```python
from build123d import *

# Parameters (mm, degrees)
BASPROSKE_W             = 7
BASPROSKE_H             = 10.5
TOOTHCUT_DEPTH          = 17.416455159
TEETHCUTS_COUNT         = 12
TEETHCUTS_ANGLE         = 330
BORSKE_R                = 2.5
BORE_DEPTH              = 50.0000508
CROQUIS2_R              = 2.91
CORTAR_EXTRUIR1_DEPTH   = 11
CROQUIS3_R              = 3.252376505
CROQUIS3_R_2            = 1.9
SALIENTE_EXTRUIR2_DEPTH = 0.79


with BuildPart() as part:
    # BasProSke → Base-Revolve (revolve)
    with BuildSketch(Plane(origin=(0, 0, 0), x_dir=(1, 0, 0), z_dir=(0, 1, 0)), mode=Mode.PRIVATE) as base_revolve_sk:
        with Locations((3.5, 5.25)):
            Rectangle(BASPROSKE_W, BASPROSKE_H)
    revolve(base_revolve_sk.sketch.rotate(Axis((-10, 0, 0), (1, 0, 0)), 180), axis=Axis((-10, 0, 0), (1, 0, 0)))

    # TooCutSke → ToothCut (cut, through all)
    with BuildSketch(Plane(origin=(0, 0, 0), x_dir=(0, 0, -1), z_dir=(1, 0, 0))):
        with BuildLine():
            ThreePointArc((0.837751456, 7.074570552), (0, 7.124), (-0.837751456, 7.074570552))
            ThreePointArc((-0.837751456, 7.074570552), (-1.245380016, 8.868946541), (-2.486473743, 10.227487154))
            ThreePointArc((-2.486473743, 10.227487154), (0, 10.5254), (2.486473743, 10.227487154))
            ThreePointArc((2.486473743, 10.227487154), (1.245380016, 8.868946541), (0.837751456, 7.074570552))
        make_face()
    toothcut = extrude(amount=TOOTHCUT_DEPTH, mode=Mode.SUBTRACT)

    # TeethCuts: ToothCut ×12 about axis
    teethcuts_axis = Axis((-10, 0, 0), (1, 0, 0))
    for i in range(1, TEETHCUTS_COUNT):
        add(toothcut.rotate(teethcuts_axis, i * TEETHCUTS_ANGLE / (TEETHCUTS_COUNT - 1)), mode=Mode.SUBTRACT)

    # BorSke → Bore (cut, symmetric)
    with BuildSketch(Plane(origin=(0, 0, 0), x_dir=(0, 0, -1), z_dir=(1, 0, 0))):
        with Locations(Location((0, 0, 0), (0, 0, 180))):
            Circle(BORSKE_R)
    extrude(amount=BORE_DEPTH, both=True, mode=Mode.SUBTRACT)

    # Croquis2 → Cortar-Extruir1 (cut)
    with BuildSketch(Plane.ZY):
        Circle(CROQUIS2_R)
    extrude(amount=-CORTAR_EXTRUIR1_DEPTH, mode=Mode.SUBTRACT)

    # Croquis3 → Saliente-Extruir2 (add, symmetric)
    with BuildSketch(Plane(origin=(1, 0, 0), x_dir=(0, 0, -1), z_dir=(1, 0, 0))):
        Circle(CROQUIS3_R)
        with Locations(Location((0, 0, 0), (0, 0, 180))):
            Circle(CROQUIS3_R_2, mode=Mode.SUBTRACT)
    extrude(amount=SALIENTE_EXTRUIR2_DEPTH, both=True)


solid = part.part
```
For this review, take the finished solid that the model builds, in its own axes (mm). Round coordinates to 2 decimals unless told otherwise and drop trailing zeros. Write each loop counter-clockwise with the first axis right and the second up, starting at its lowest first coordinate (ties: lowest second). Pieces come first, ordered by that corner, then holes. Notation, with made-up numbers: (79, 86) -> (94, 86) arc R11 ccw to (94, 92) -> close; hole circle Ø3 at (18, 1.25). An arc over 180 degrees is marked (long way). One line per question, with ' | ' between items. Start each with the question number.
1) Wall thickness on line 1 along Y through (x, z) = (1.35, 0); line 2 along Y through (x, z) = (0.1, 0); line 3 along Z through (x, y) = (5.5, 6.25): over which ranges is each line inside the solid? List them lowest first.
2) Add section A-A (z = 0). Write out the cut boundary in (x, y).
3) Mouldability with a two-part tool opening along Z and no side actions: class faces 1 (the flat face through (7, -2.4, 2.4)), 2 (the cylindrical face through (4.359, 2.885, -0.379)), 3 (the cylindrical face through (3.451, -5.477, 7.035)) as +Z half, -Z half, draft (parallel to the pull), parting line (faces both ways), or undercut.
4) Add section C-C (z = -4). Write out the cut boundary in (x, y), and give its area (3 significant figures).
5) For pin 1 Ø1 at (y, z) = (-6.5, 6) entering from -X; pin 2 Ø1.5 at (x, y) = (2.5, -3.5) entering from +Z; pin 3 Ø4.5 at (y, z) = (0, 0) entering from +X; pin 4 Ø1.5 at (x, y) = (5, 7) entering from +Z, all flat-tipped, find the tip position at first contact; note any pin that passes through.
Reported:
1) line 1: y = -7.12 to -1.9, 1.9 to 7.12 | line 2: y = -7.12 to -2.91, 2.91 to 7.12 | line 3: z = -7.42 to -4.62, -3.42 to 3.42, 4.62 to 7.42
2) outline: (0, -7.12) -> (7, -7.12) -> (7, -2.91) -> (1.79, -2.91) -> (1.79, -1.9) -> (0.21, -1.9) -> (0.21, -2.91) -> (0, -2.91) -> close; (0, 2.91) -> (0.21, 2.91) -> (0.21, 1.9) -> (1.79, 1.9) -> (1.79, 2.91) -> (7, 2.91) -> (7, 7.12) -> (0, 7.12) -> close
3) face 1: draft | face 2: undercut | face 3: +Z half
4) outline: (0, -5.9) -> (7, -5.9) -> (7, 5.9) -> (0, 5.9) -> close | area: 82.5 mm²
5) pin 1: stops at x = 0 | pin 2: stops at z = 10.13 | pin 3: stops at x = 1.79 | pin 4: stops at z = 7.61
